from build123d import *

# Parameters (mm, degrees)
SKETCH1_R           = 10.1
BOSS_EXTRUDE1_DEPTH = 10
SKETCH2_R           = 16.1
SKETCH2_R_2         = 10.1
BOSS_EXTRUDE2_DEPTH = 20
FILLET1_R           = 5
CUT_EXTRUDE1_DEPTH  = 20


with BuildPart() as part:
    # Sketch1 → Boss-Extrude1 (new body)
    with BuildSketch(Plane(origin=(0, 0, 0), x_dir=(0, 0, -1), z_dir=(1, 0, 0))):
        Polygon((14.60696181, 25.3), (-14.60696181, 25.3), (-29.213923621, 0), (-14.60696181, -25.3), (14.60696181, -25.3), (29.213923621, 0), align=None)
        Circle(SKETCH1_R, mode=Mode.SUBTRACT)
    extrude(amount=BOSS_EXTRUDE1_DEPTH)

    # Sketch2 → Boss-Extrude2 (add)
    with BuildSketch(Plane(origin=(10, 0, 0), x_dir=(0, 0, -1), z_dir=(1, 0, 0))):
        Circle(SKETCH2_R)
        Circle(SKETCH2_R_2, mode=Mode.SUBTRACT)
    extrude(amount=BOSS_EXTRUDE2_DEPTH)

    # Fillet1
    fillet1_edges = [part.edges().sort_by_distance(p)[0] for p in [
        (10, 0, 16.1),
    ]]
    fillet(fillet1_edges, radius=FILLET1_R)

    # Sketch3 → Cut-Extrude1 (cut)
    with BuildSketch(Plane(origin=(0, 0, 0), x_dir=(1, 0, 0), z_dir=(0, 1, 0))):
        with BuildLine():
            ThreePointArc((21, 0), (22.5, -1.5), (24, 0))
            Line((24, 0), (21, 0))
        make_face()
        with BuildLine():
            Line((21, 0), (24, 0))
            ThreePointArc((24, 0), (22.5, 1.5), (21, 0))
        make_face()
    extrude(amount=-CUT_EXTRUDE1_DEPTH, mode=Mode.SUBTRACT)


solid = part.part
Design review of the part built by this model. Coordinates are the model's own, in mm. A direction names the side the tool comes from. Give positions to 0.01 mm unless a question says otherwise; leave off trailing zeros. Order: outer loops, then holes, each group sorted by start corner. A loop starts at its lowest first (then second) coordinate and runs counter-clockwise, first axis right, second up. Notation, with made-up numbers: (38, 86) - (83, 86) arc R13 ccw to (83, 102) - close; hole circle Ø7 at (-8, -9). An arc over 180 degrees is marked (long way). Write item = value, one per line. Start each with the question number.
Q1. We need section A-A on z = 0. State the section outline as (x, y) points, plus the area to 3 significant figures.
Q2. Tool access review of faces 5 (the face through (5, -25.3, 0)), 6 (the face through (10, 21, -6)): name each direction out of +Z, -Z, +X, -X, +Y, -Y from which nothing blocks a thin tool from reaching the whole face with its end or side.
Q3. Clearance check with a flat-ended pin moving along its axis: pin 1 Ø4 at (x, z) = (22.5, 0) entering from -Y. State where the tip first meets the part, or that it passes through.
Q4. Mouldability with a two-part tool opening along Z and no side actions: class faces 1 (the face through (4.93, -12.827, -21.808)), 2 (the face through (14.79, 3.034, -9.634)), 3 (the face through (21, -13, 0)), 4 (the face through (4.93, 12.827, 21.808)) as released by +Z, released by -Z, zero draft, split by the parting line, or undercut.
Q5. To check wall thickness, follow L1, parallel to Y at x = 7, z = 0; L2, parallel to X at y = -11, z = 0; L3, parallel to Z at x = 23, y = 7.5. State the ranges of each line that lie inside material, in increasing order. Write a range as from..to.
Q6. We need section B-B on x = 3. State the section outline as (y, z) points, plus the area to 3 significant figures.
Q7. We need section D-D on x = 27. State the section outline as (y, z) points.
Q8. We need section C-C on z = 24. State the section outline as (x, y) points, plus the area to 3 significant figures.
Working result:
q1.outline = (0, -25.3) - (10, -25.3) - (10, -21.1) arc R5 cw to (15, -16.1) - (21, -16.1) - (21, -10.1) - (0, -10.1) - close; (0, 10.1) - (30, 10.1) - (30, 16.1) - (15, 16.1) arc R5 cw to (10, 21.1) - (10, 25.3) - (0, 25.3) - close; (24, -16.1) - (30, -16.1) - (30, -10.1) - (24, -10.1) - close
q1.area = 537 mm²
q2.face_5 = +Z, -Z, +X, -X, -Y
q2.face_6 = +X
q3.pin_1 = -16.1
q4.face_1 = released by -Z
q4.face_2 = undercut
q4.face_3 = undercut
q4.face_4 = released by +Z
q5.L1 = -25.3..-10.1, 10.1..25.3
q5.L2 = 0..21, 24..30
q5.L3 = -14.25..-6.76, 6.76..14.25
q6.outline = (-25.3, -14.61) - (0, -29.21) - (25.3, -14.61) - (25.3, 14.61) - (0, 29.21) - (-25.3, 14.61) - close; hole circle Ø20.2 at (0, 0)
q6.area = 1,900 mm²
q7.outline = circle Ø32.2 at (0, 0); hole circle Ø20.2 at (0, 0)
q8.outline = (0, -9.03) - (10, -9.03) - (10, 9.03) - (0, 9.03) - close
q8.area = 181 mm²
